from build123d import *

# Parameters (mm, degrees)
RESSALTO_EXTRUS_O1_DEPTH = 2.5


with BuildPart() as part:
    # Esboço1 → Ressalto-extrusão1 (new body)
    with BuildSketch(Plane.XY):
        with BuildLine():
            Line((53.368768098, -72.405467359), (-27.631231902, -72.405467359))
            ThreePointArc((-27.631231902, -72.405467359), (-29.398998855, -73.137700406), (-30.131231902, -74.905467359))
            Line((-30.131231902, -74.905467359), (-30.131231902, -98.905467359))
            ThreePointArc((-30.131231902, -98.905467359), (-29.398998855, -100.673234312), (-27.631231902, -101.405467359))
            Line((-27.631231902, -101.405467359), (-26.934280418, -101.405467359))
            Line((-26.934280418, -101.405467359), (-26.934280418, -86.405467359))
            Line((-26.934280418, -86.405467359), (-24.231231902, -86.405467359))
            Line((-24.231231902, -86.405467359), (-24.231231902, -101.405467359))
            Line((-24.231231902, -101.405467359), (-10.131231902, -101.405467359))
            Line((-10.131231902, -101.405467359), (-10.131231902, -96.405467359))
            Line((-10.131231902, -96.405467359), (-7.631231902, -96.405467359))
            Line((-7.631231902, -96.405467359), (-7.631231902, -101.405467359))
            Line((-7.631231902, -101.405467359), (33.368768098, -101.405467359))
            Line((33.368768098, -101.405467359), (33.368768098, -96.405467359))
            Line((33.368768098, -96.405467359), (35.868768098, -96.405467359))
            Line((35.868768098, -96.405467359), (35.868768098, -101.405467359))
            Line((35.868768098, -101.405467359), (49.968768098, -101.405467359))
            Line((49.968768098, -101.405467359), (49.968768098, -86.405467359))
            Line((49.968768098, -86.405467359), (52.671816614, -86.405467359))
            Line((52.671816614, -86.405467359), (52.671816614, -101.405467359))
            Line((52.671816614, -101.405467359), (53.368768098, -101.405467359))
            ThreePointArc((53.368768098, -101.405467359), (55.136535051, -100.673234312), (55.868768098, -98.905467359))
            Line((55.868768098, -98.905467359), (55.868768098, -74.905467359))
            ThreePointArc((55.868768098, -74.905467359), (55.136535051, -73.137700406), (53.368768098, -72.405467359))
        make_face()
    extrude(amount=RESSALTO_EXTRUS_O1_DEPTH)


solid = part.part
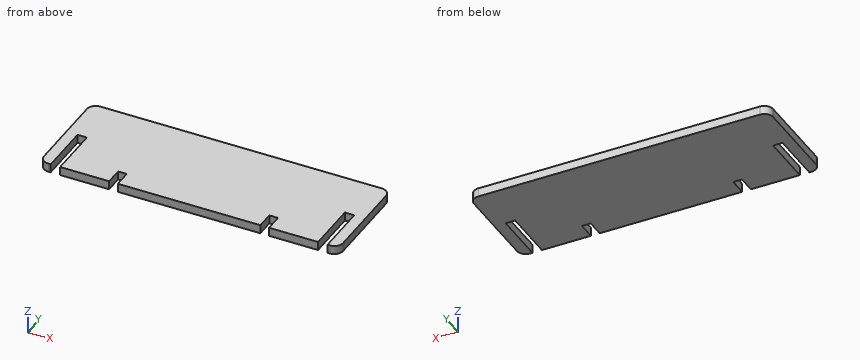
Work out the finished part from the listing and answer in its coordinate system (mm). Give positions to 0.01 mm unless a question says otherwise; leave off trailing zeros. Loops run counter-clockwise (first coordinate to the right, second up) from the corner with the lowest first, then second, coordinate; pieces in that order, holes last. Notation, with made-up numbers: (68.5, 35) -> (88.5, 35) arc R20 cw to (88.5, 63) -> close; hole circle Ø4 at (42.5, 27). An arc over 180 degrees is marked (long way). Use a Markdown table: item, result. Add a question column.
1. Flat-ended cylindrical pins translate along their axes: pin 1 Ø0.8 at (x, z) = (-8.5, 2) entering from -Y; pin 2 Ø0.8 at (y, z) = (-99.5, 1.5) entering from -X; pin 3 Ø0.8 at (x, z) = (51.5, 1) entering from -Y. Find the tip coordinate at first contact, or state that the pin passes through.
2. Section B-B on x = -9 is taken. Determine the outline of the cut face in (y, z), and give its area (3 significant figures).
3. Find the intervals of material crossed by probe 1 along X at (y, z) = (-92, 0.1); probe 2 along X at (y, z) = (-97, 2.15); probe 3 along Y at (x, z) = (-9, 1.05), in increasing order.
4. Section A-A on z = 2 is taken. Determine the outline of the cut face in (x, y), and give its area (3 significant figures).
Results below:
| question | item | result |
|---|---|---|
| 1 | pin 1 | stops at y = -96.41 |
| 1 | pin 2 | stops at x = -30.12 |
| 1 | pin 3 | stops at y = -86.41 |
| 2 | outline | (-96.41, 0) -> (-72.41, 0) -> (-72.41, 2.5) -> (-96.41, 2.5) -> close |
| 2 | area | 60.0 mm^2 |
| 3 | probe 1 | x = -30.13 to -26.93, -24.23 to 49.97, 52.67 to 55.87 |
| 3 | probe 2 | x = -30.13 to -26.93, -24.23 to -10.13, -7.63 to 33.37, 35.87 to 49.97, 52.67 to 55.87 |
| 3 | probe 3 | y = -96.41 to -72.41 |
| 4 | outline | (-30.13, -98.91) arc R2.5 ccw to (-27.63, -101.41) -> (-26.93, -101.41) -> (-26.93, -86.41) -> (-24.23, -86.41) -> (-24.23, -101.41) -> (-10.13, -101.41) -> (-10.13, -96.41) -> (-7.63, -96.41) -> (-7.63, -101.41) -> (33.37, -101.41) -> (33.37, -96.41) -> (35.87, -96.41) -> (35.87, -101.41) -> (49.97, -101.41) -> (49.97, -86.41) -> (52.67, -86.41) -> (52.67, -101.41) -> (53.37, -101.41) arc R2.5 ccw to (55.87, -98.91) -> (55.87, -74.91) arc R2.5 ccw to (53.37, -72.41) -> (-27.63, -72.41) arc R2.5 ccw to (-30.13, -74.91) -> close |
| 4 | area | 2,380 mm^2 |
